from build123d import *
from build123d.topology import SkipClean

# Parameters (mm, degrees)
SKETCH1_R                = 22.225
SKETCH1_R_2              = 15.875
BOSS_EXTRUDE1_DEPTH      = 3.175
BOSS_EXTRUDE2_DEPTH      = 3.175
F_0_257_DIAMETER_HOLE1_D = 6.5278
SKETCH6_W                = 65.552410467
SKETCH6_H                = 82.171101747
CUT_EXTRUDE2_DEPTH       = 86.310457973
BOSS_EXTRUDE3_DEPTH      = 3.175
SKETCH12_R               = 2.15265
CUT_EXTRUDE4_DEPTH       = 80.867912855
SKETCH13_R               = 5.8039
SKETCH13_R_2             = 3.2639
BOSS_EXTRUDE4_DEPTH      = 9.525
MIRROR2_START            = -3.175
MIRROR2_OUTLINE_R        = 3.2639
MIRROR2_DEPTH            = 1.0223499
MIRROR2_START_2          = 12.081931798
MIRROR2_2_OUTLINE_W      = 2.1526501
MIRROR2_2_OUTLINE_H      = 12.8778
MIRROR2_2_DEPTH          = 70.221427729
MIRROR2_START_3          = 10.16
MIRROR2_3_DEPTH          = 11.111840348
MIRROR2_4_DEPTH          = 6.35
MIRROR2_START_4          = -2.1526501
MIRROR2_5_OUTLINE_R      = 3.2639
MIRROR2_5_DEPTH          = 2.1526501
FILLET5_R                = 2.54


with BuildPart() as part:
    # Sketch1 → Boss-Extrude1 (new body)
    with BuildSketch(Plane(origin=(0, 0, 0), x_dir=(1, 0, 0), z_dir=(0, 1, 0))):
        with Locations(Location((0, 0, 0), (0, 0, 270))):
            Circle(SKETCH1_R)
        with Locations(Location((0, 0, 0), (0, 0, 270))):
            Circle(SKETCH1_R_2, mode=Mode.SUBTRACT)
    extrude(amount=BOSS_EXTRUDE1_DEPTH)

    # Sketch2 → Boss-Extrude2 (add)
    with BuildSketch(Plane(origin=(0, 3.175, 0), x_dir=(1, 0, 0), z_dir=(0, 1, 0))):
        with BuildLine():
            Line((75.953359527, -6.4389), (38.518839527, -6.4389))
            Line((38.518839527, -6.4389), (17.590769706, -6.4389))
            Line((17.590769706, -6.4389), (17.590769706, 6.4389))
            Line((17.590769706, 6.4389), (38.518839527, 6.4389))
            Line((38.518839527, 6.4389), (75.953359527, 6.4389))
            ThreePointArc((75.953359527, 6.4389), (80.443487588, 4.579028061), (82.303359527, 0.0889))
            Line((82.303359527, 0.0889), (82.303359527, -0.0889))
            ThreePointArc((82.303359527, -0.0889), (80.443487588, -4.579028061), (75.953359527, -6.4389))
        make_face()
    extrude(amount=-BOSS_EXTRUDE2_DEPTH)

    # F (0.257) Diameter Hole1 (through all)
    with Locations(Plane(origin=(0, 3.175, 0), x_dir=(1, 0, 0), z_dir=(0, 1, 0))):
        with Locations((69.85, 0)):
            Hole(F_0_257_DIAMETER_HOLE1_D / 2)

    # Sketch6 → Cut-Extrude2 (cut, through all)
    with BuildSketch(Plane(origin=(0, 3.175, 0), x_dir=(1, 0, 0), z_dir=(0, 1, 0))):
        with Locations((-22.616205234, -1.153387837)):
            Rectangle(SKETCH6_W, SKETCH6_H)
    extrude(amount=-CUT_EXTRUDE2_DEPTH, mode=Mode.SUBTRACT)

    # Sketch9 → Boss-Extrude3 (add)
    with BuildSketch(Plane(origin=(0, 3.175, 0), x_dir=(1, 0, 0), z_dir=(0, 1, 0))):
        Polygon((10.16, 19.766765669), (10.16, 45.166765669), (16.51, 45.166765669), (16.51, 14.878525633), align=None)
    boss_extrude3 = extrude(amount=-BOSS_EXTRUDE3_DEPTH)

    # Mirror1: Boss-Extrude3 across plane
    add(boss_extrude3.mirror(Plane.XY))

    # Sketch12 → Cut-Extrude4 (cut, through all)
    with BuildSketch(Plane(origin=(16.51, 0, 0), x_dir=(0, 0, -1), z_dir=(1, 0, 0))):
        with Locations((38.1, 0)):
            Circle(SKETCH12_R)
        with Locations((-38.1, 0)):
            Circle(SKETCH12_R)
    extrude(amount=-CUT_EXTRUDE4_DEPTH, mode=Mode.SUBTRACT)

    # Sketch13 → Boss-Extrude4 (add)
    with SkipClean():  # the faces are left unmerged after this step: merging them gives an invalid solid
        with BuildSketch(Plane(origin=(0, 3.175, 0), x_dir=(1, 0, 0), z_dir=(0, 1, 0))):
            with Locations(Location((69.85, 0, 0), (0, 0, 90))):
                Circle(SKETCH13_R)
            with Locations(Location((69.85, 0, 0), (0, 0, 270))):
                Circle(SKETCH13_R_2, mode=Mode.SUBTRACT)
        extrude(amount=BOSS_EXTRUDE4_DEPTH)



with BuildPart() as body_2:
    # Mirror2: read off the stored shape, not the designer's step
    # Mirror2 outline → Mirror2 (new body)
    with BuildSketch(Plane(origin=(0, 0, 0), x_dir=(1, 0, 0), z_dir=(0, 1, 0)).offset(MIRROR2_START)):
        with BuildLine():
            Line((10.16, 45.166765669), (10.16, 12.197951672))
            ThreePointArc((10.16, 12.197951672), (15.875, 0), (10.16, -12.197951672))
            Line((10.16, -12.197951672), (10.16, -45.166765669))
            Line((10.16, -45.166765669), (16.51, -45.166765669))
            Line((16.51, -45.166765669), (16.51, -14.878525633))
            ThreePointArc((16.51, -14.878525633), (19.356489486, -10.921398252), (21.271840348, -6.4389))
            Line((21.271840348, -6.4389), (75.953359527, -6.4389))
            ThreePointArc((75.953359527, -6.4389), (80.443487588, -4.579028061), (82.303359527, -0.0889))
            Line((82.303359527, -0.0889), (82.303359527, 0.0889))
            ThreePointArc((82.303359527, 0.0889), (80.443487588, 4.579028061), (75.953359527, 6.4389))
            Line((75.953359527, 6.4389), (21.271840348, 6.4389))
            ThreePointArc((21.271840348, 6.4389), (19.356489486, 10.921398252), (16.51, 14.878525633))
            Line((16.51, 14.878525633), (16.51, 45.166765669))
            Line((16.51, 45.166765669), (10.16, 45.166765669))
        make_face()
        with Locations((69.85, 0)):
            Circle(MIRROR2_OUTLINE_R, mode=Mode.SUBTRACT)
    extrude(amount=MIRROR2_DEPTH)


with BuildPart() as part_1:
    with SkipClean():  # the faces are left unmerged after this step: merging them gives an invalid solid
        add(part.part)

        add(body_2.part)  # Mirror2 2 merges body 2
        # Mirror2 2 outline → Mirror2 2 (add)
        with BuildSketch(Plane.YZ.offset(MIRROR2_START_2)):
            with Locations((-1.07632505, 0)):
                Rectangle(MIRROR2_2_OUTLINE_W, MIRROR2_2_OUTLINE_H)
        extrude(amount=MIRROR2_2_DEPTH)

    # Mirror2 3 outline → Mirror2 3 (add)
    with SkipClean():  # the faces are left unmerged after this step: merging them gives an invalid solid
        with BuildSketch(Plane.YZ.offset(MIRROR2_START_3)):
            with BuildLine():
                Line((0, -6.4389), (-2.1526501, -6.4389))
                Line((-2.1526501, -6.4389), (-2.15265, -38.1))
                ThreePointArc((-2.15265, -38.1), (-1.522153413, -36.577846587), (0, -35.94735))
                Line((0, -35.94735), (0, -6.4389))
            make_face()
            with BuildLine():
                Line((-2.15265, 38.1), (-2.1526501, 6.4389))
                Line((-2.1526501, 6.4389), (0, 6.4389))
                Line((0, 6.4389), (0, 35.94735))
                ThreePointArc((0, 35.94735), (-1.522153413, 36.577846587), (-2.15265, 38.1))
            make_face()
        extrude(amount=MIRROR2_3_DEPTH)

    # Mirror2 4 outline → Mirror2 4 (add)
    with SkipClean():  # the faces are left unmerged after this step: merging them gives an invalid solid
        with BuildSketch(Plane.YZ.offset(MIRROR2_START_3)):
            with BuildLine():
                ThreePointArc((0, -40.25265), (-1.522153413, -39.622153413), (-2.15265, -38.1))
                Line((-2.15265, -38.1), (-2.1526501, -45.166765669))
                Line((-2.1526501, -45.166765669), (0, -45.166765669))
                Line((0, -45.166765669), (0, -40.25265))
            make_face()
            with BuildLine():
                Line((-2.1526501, 45.166765669), (-2.15265, 38.1))
                ThreePointArc((-2.15265, 38.1), (-1.522153413, 39.622153413), (0, 40.25265))
                Line((0, 40.25265), (0, 45.166765669))
                Line((0, 45.166765669), (-2.1526501, 45.166765669))
            make_face()
        extrude(amount=MIRROR2_4_DEPTH)

    # Mirror2 5 outline → Mirror2 5 (cut)
    with BuildSketch(Plane(origin=(0, 0, 0), x_dir=(1, 0, 0), z_dir=(0, 1, 0)).offset(MIRROR2_START_4)):
        with BuildLine():
            Line((16.51, 40), (16.51, 14.878525633))
            ThreePointArc((16.51, 14.878525633), (19.356489486, 10.921398252), (21.271840348, 6.4389))
            Line((21.271840348, 6.4389), (21.271840348, 40))
            Line((21.271840348, 40), (16.51, 40))
        make_face()
        with BuildLine():
            Line((82.303359527, 6.4389), (75.953359527, 6.4389))
            ThreePointArc((75.953359527, 6.4389), (80.443487588, 4.579028061), (82.303359527, 0.0889))
            Line((82.303359527, 0.0889), (82.303359527, 6.4389))
        make_face()
        with BuildLine():
            Line((10.16, 6.4389), (12.081931798, 6.4389))
            Line((12.081931798, 6.4389), (12.081931798, -6.4389))
            Line((12.081931798, -6.4389), (10.16, -6.4389))
            Line((10.16, -6.4389), (10.16, -12.197951672))
            ThreePointArc((10.16, -12.197951672), (15.875, 0), (10.16, 12.197951672))
            Line((10.16, 12.197951672), (10.16, 6.4389))
        make_face()
        with BuildLine():
            Line((82.303359527, -6.4389), (82.303359527, -0.0889))
            ThreePointArc((82.303359527, -0.0889), (80.443487588, -4.579028061), (75.953359527, -6.4389))
            Line((75.953359527, -6.4389), (82.303359527, -6.4389))
        make_face()
        with BuildLine():
            Line((21.271840348, -40), (21.271840348, -6.4389))
            ThreePointArc((21.271840348, -6.4389), (19.356489486, -10.921398252), (16.51, -14.878525633))
            Line((16.51, -14.878525633), (16.51, -40))
            Line((16.51, -40), (21.271840348, -40))
        make_face()
        with Locations((69.85, 0)):
            Circle(MIRROR2_5_OUTLINE_R)
    extrude(amount=MIRROR2_5_DEPTH, mode=Mode.SUBTRACT)

    # Fillet5
    fillet5_edges = [part_1.edges().sort_by_distance(p)[0] for p in [
        (13.335, -3.175, -45.166765669),
        (13.335, -3.175, 45.166765669),
        (13.335, 3.175, -45.166765669),
        (10.16, 1.5875, -45.166765669),
        (16.51, 1.5875, -45.166765669),
        (13.335, 3.175, 45.166765669),
        (16.51, 1.5875, 45.166765669),
        (10.16, 1.5875, 45.166765669),
    ]]
    fillet(fillet5_edges, radius=FILLET5_R)


solid = part_1.part
The model under review builds one solid part; all positions refer to its coordinate system, in mm. A direction names the side the tool comes from. Give positions to 0.01 mm unless a question says otherwise; leave off trailing zeros. Write each loop counter-clockwise with the first axis right and the second up, starting at its lowest first coordinate (ties: lowest second). Pieces come first, ordered by that corner, then holes.
1. Add section D-D, the plane x = 19.5. Write out the cut boundary in (y, z) (3 decimals).
2. Add section C-C, the plane z = 9. Write out the cut boundary in (x, y) (3 decimals), plus the area to 3 significant figures.
3. Add section B-B, the plane y = 11. Write out the cut boundary in (x, z), plus the area to 3 significant figures.
4. For P1, Ø21.5, axis at x = 39.5, z = 4.5, coming from the +Y side (3 decimals); P2, Ø4, axis at x = 43, y = 0.5, coming from the +Z side; P3, Ø5, axis at x = 62, y = -1.5, coming from the -Z side; P4, Ø7.5, axis at x = 69.85, z = 0, coming from the -Y side (3 decimals), all flat-tipped, find the tip position at first contact; note any pin that passes through.
5. Add section A-A, the plane x = 69.85. Write out the cut boundary in (y, z) (3 decimals), plus the area to 3 significant figures.
6. Wall thickness on L1, parallel to Z at x = 69.85, y = 9.25; L2, parallel to Z at x = 69.85, y = -0.95; L3, parallel to X at y = 5.75, z = 0: over which ranges is each line inside the solid? List them lowest first.
7. Tool access review of faces 1 (the flat face through (49, 0, 6.439)), 2 (the cylindrical face through (75.516, 7.871, 1.258)), 3 (the flat face through (48, 0, -6.439)): name each direction out of +Z, -Z, +X, -X, +Y, -Y from which nothing blocks a thin tool from reaching the whole face with its end or side.
Worked answers:
1. outline: (-3.175, -10.663) - (3.175, -10.663) - (3.175, 10.663) - (-3.175, 10.663) - close
2. outline: (13.077, -3.175) - (20.321, -3.175) - (20.321, 3.175) - (13.077, 3.175) - close
2. area: 46.0 mm2
3. outline: circle Ø11.61 at (69.85, 0); hole circle Ø6.53 at (69.85, 0)
3. area: 72.4 mm2
4. P1: stops at y = 3.175
4. P2: stops at z = 6.44
4. P3: stops at z = -6.44
4. P4: stops at y = -3.175
5. outline: (-3.175, -6.439) - (3.175, -6.439) - (3.175, -5.804) - (12.7, -5.804) - (12.7, -3.264) - (-3.175, -3.264) - close; (-3.175, 3.264) - (12.7, 3.264) - (12.7, 5.804) - (3.175, 5.804) - (3.175, 6.439) - (-3.175, 6.439) - close
5. area: 88.7 mm2
6. L1: z = -5.8 to -3.26, 3.26 to 5.8
6. L2: z = -6.44 to -3.26, 3.26 to 6.44
6. L3: x = 64.05 to 66.59, 73.11 to 75.65
7. face 1: +Z, +X, +Y, -Y
7. face 2: +Y
7. face 3: -Z, +X, +Y, -Y
